from build123d import *

# Parameters (mm, degrees)
SKETCH1_R               = 6.67
BOSS_EXTRUDE1_DEPTH     = 0.15
CHAMFER1_SIZE           = 0.3
CHAMFER1_SIZE2          = 0.05
CHAMFER2_SIZE           = 0.05
CHAMFER2_SIZE2          = 0.3
SKETCH2_R               = 0.3105
CUT_EXTRUDE1_DEPTH      = 1.15
CUT_EXTRUDE1_DEPTH_BACK = 1.15
CUT_EXTRUDE2_DEPTH      = 1.15
CIRPATTERN1_COUNT       = 3


with BuildPart() as part:
    # Sketch1 → Boss-Extrude1 (new body, symmetric)
    with BuildSketch(Plane.XY):
        Circle(SKETCH1_R)
    extrude(amount=BOSS_EXTRUDE1_DEPTH, both=True)

    # Chamfer1
    chamfer1_edges = [part.edges().sort_by_distance(p)[0] for p in [
        (-6.67, 0, -0.15),
    ]]
    chamfer1_side = [part.faces().sort_by_distance(p)[0] for p in [
        (0, 0, -0.15),
    ]]
    chamfer(chamfer1_edges, length=CHAMFER1_SIZE, length2=CHAMFER1_SIZE2, reference=chamfer1_side[0])

    # Chamfer2
    chamfer2_edges = [part.edges().sort_by_distance(p)[0] for p in [
        (-6.67, 0, 0.15),
    ]]
    chamfer2_side = [part.faces().sort_by_distance(p)[0] for p in [
        (-6.67, 0, 0.025),
    ]]
    chamfer(chamfer2_edges, length=CHAMFER2_SIZE, length2=CHAMFER2_SIZE2, reference=chamfer2_side[0])

    # Sketch2 → Cut-Extrude1 (cut, two sides)
    with BuildSketch(Plane.XY) as cut_extrude1_sk:
        Circle(SKETCH2_R)
    extrude(amount=CUT_EXTRUDE1_DEPTH, mode=Mode.SUBTRACT)
    extrude(cut_extrude1_sk.sketch, amount=-CUT_EXTRUDE1_DEPTH_BACK, mode=Mode.SUBTRACT)

    # Sketch3 → Cut-Extrude2 (cut, symmetric)
    with BuildSketch(Plane.XY):
        with BuildLine():
            ThreePointArc((1.039913882, 6.010705376), (1.065211247, 0.615), (5.725380491, -2.104760848))
            ThreePointArc((5.725380491, -2.104760848), (5.282754963, 3.05), (1.039913882, 6.010705376))
        make_face()
    cut_extrude2 = extrude(amount=CUT_EXTRUDE2_DEPTH, both=True, mode=Mode.SUBTRACT)

    # CirPattern1: Cut-Extrude2 ×3 about axis
    cirpattern1_axis = Axis((0, 0, 0), (0, 0, 1))
    for i in range(1, CIRPATTERN1_COUNT):
        add(cut_extrude2.rotate(cirpattern1_axis, i * 360 / CIRPATTERN1_COUNT), mode=Mode.SUBTRACT)


solid = part.part
Work out the finished part from the listing and answer in its coordinate system (mm). Round coordinates to 2 decimals unless told otherwise and drop trailing zeros. Write each loop counter-clockwise with the first axis right and the second up, starting at its lowest first coordinate (ties: lowest second). Pieces come first, ordered by that corner, then holes. Notation, with made-up numbers: M 75.25,29.25 L 104.25,29.25 A14 ccw 104.25,38.25 Z; hole C -36,82.25 d2. An arc over 180 degrees is marked long. Use a Markdown table: item, result.
1) Determine the mould class of faces 1 (the face through (0, 1, -0.15)), 2 (the face through (1.03, 0.68, 0)) for opening direction X: pulls with the +X half, pulls with the -X half, needs draft (parallel to the pull), parting line crosses it, or undercut.
Taken from the geometry:
| item | result |
|---|---|
| face 1 | needs draft |
| face 2 | undercut |
2) The part is cut by section C-C on y = 5.5. State how many separate pieces and enclosed holes the cut face has, plus the area to 3 significant figures.
Taken from the geometry:
| item | result |
|---|---|
| separate pieces | 3 |
| enclosed holes | 0 |
| area | 1.10 mm2 |
3) The part is cut by section A-A on x = 0. Give the vertices of the cut face in (y, z), plus the area to 3 significant figures.
Taken from the geometry:
| item | result |
|---|---|
| outline | M -6.67,-0.1 L -6.37,-0.15 L -6.1,-0.15 L -6.1,0.15 L -6.37,0.15 L -6.67,0.1 Z; M -1.23,-0.15 L -0.31,-0.15 L -0.31,0.15 L -1.23,0.15 Z; M 0.31,-0.15 L 6.37,-0.15 L 6.67,-0.1 L 6.67,0.1 L 6.37,0.15 L 0.31,0.15 Z |
| area | 2.32 mm2 |
4) A flat-ended cylindrical pin translates along its axis: pin 1 (6 mm diameter, centred on x = 4.5, y = -1.5, fed in from +Z). Find the tip coordinate at first contact, or state that the pin passes through.
Taken from the geometry:
| item | result |
|---|---|
| pin 1 | stops at z = 0.15 |
5) The part is cut by section B-B on y = 0. Give the vertices of the cut face in (x, z).
Taken from the geometry:
| item | result |
|---|---|
| outline | M -6.67,-0.1 L -6.37,-0.15 L -6.1,-0.15 L -6.1,0.15 L -6.37,0.15 L -6.67,0.1 Z; M -1.48,-0.15 L -0.31,-0.15 L -0.31,0.15 L -1.48,0.15 Z; M 0.31,-0.15 L 1.48,-0.15 L 1.48,0.15 L 0.31,0.15 Z; M 6.1,-0.15 L 6.37,-0.15 L 6.67,-0.1 L 6.67,0.1 L 6.37,0.15 L 6.1,0.15 Z |
6) Consider line 1 (Y direction, x = 1.5, z = -0.05); line 2 (X direction, y = 2.75, z = -0.05); line 3 (X direction, y = 4.75, z = 0.05). Determine where each line is inside the solid, lowest interval first. Write a range as [from, to].
Taken from the geometry:
| item | result |
|---|---|
| line 1 | y = [-6.5, -5.91], [-1.44, -0.03], [5.91, 6.5] |
| line 2 | x = [-6.08, -5.44], [-0.37, 0.37], [5.44, 6.08] |
| line 3 | x = [-4.68, -3.83], [-0.52, 0.52], [3.83, 4.68] |
